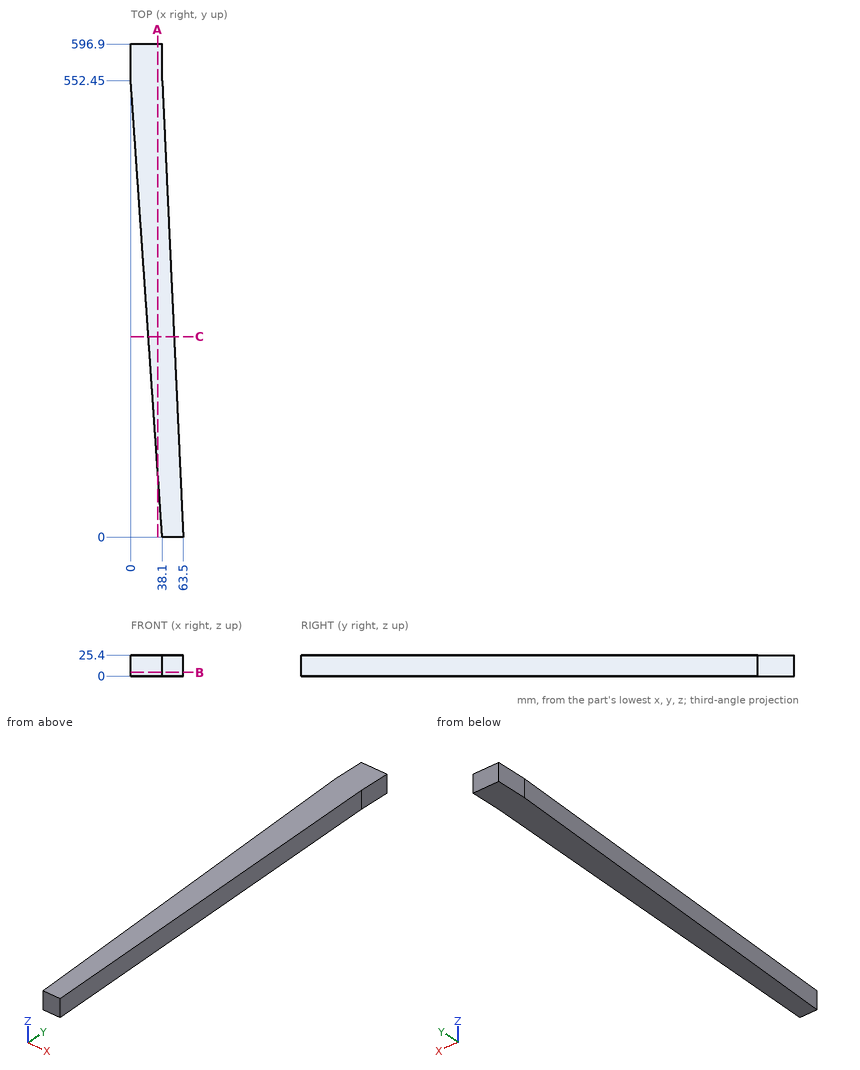
Verification items for this drawing (mm, ordinates from the low corner). Round coordinates to 2 decimals unless told otherwise and drop trailing zeros. Loops run counter-clockwise (first coordinate to the right, second up) from the corner with the lowest first, then second, coordinate; pieces in that order, holes last. Notation, with made-up numbers: (-35.5, 77) - (3.5, 77) arc R22 cw to (3.5, 95) - close; hole circle Ø1 at (-38, 55). An arc over 180 degrees is marked (long way). Answer as CSV lines item,"result". Start each with the question number.
Item 1: Section check B-B (z = 4.25). Record the boundary of the cut face in (x, y).
Item 2: Depth check by flat-ended pin: P1, Ø1.5, axis at y = 225.5, z = 5.5, coming from the +X side; P2, Ø7.5, axis at y = 579.5, z = 11, coming from the +X side; P3, Ø1, axis at y = 396.5, z = 2.5, coming from the -X side; P4, Ø1.5, axis at x = 48, y = 60, coming from the -Z side. Enter the tip coordinate at first touch or a pass-through.
Item 3: Section check A-A (x = 32.5). Record the boundary of the cut face in (y, z), and give its area (3 significant figures).
Item 4: Section check C-C (y = 242.5). Record the boundary of the cut face in (x, z).
Item 5: Scan lines: line 1 (X direction, y = 390.5, z = 4); line 2 (X direction, y = 245.5, z = 16.75). Record each from-to range of solid material in increasing order. Write a range as [from, to].
Report:
1,outline,"(0, 552.45) - (38.1, 0) - (63.5, 0) - (38.1, 552.45) - (38.1, 596.9) - (0, 596.9) - close"
2,P1,"stops at x = 53.17"
2,P2,"stops at x = 38.1"
2,P3,"stops at x = 10.72"
2,P4,"stops at z = 0"
3,outline,"(81.2, 0) - (596.9, 0) - (596.9, 25.4) - (81.2, 25.4) - close"
3,area,"13,100 mm2"
4,outline,"(21.38, 0) - (52.35, 0) - (52.35, 25.4) - (21.38, 25.4) - close"
5,line 1,"x = [11.17, 45.55]"
5,line 2,"x = [21.17, 52.21]"
